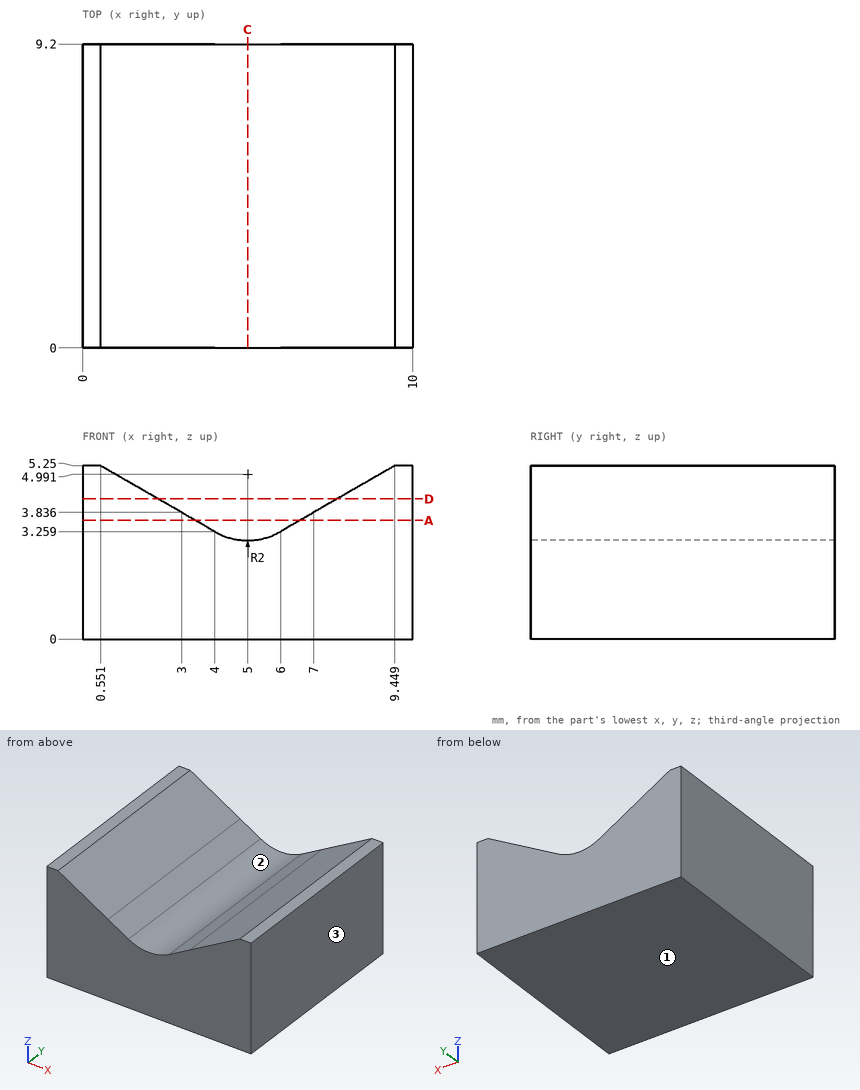
Design review of the part shown in the three views and the two pictorial views. Dimensions are in mm from the part's minimum x, y and z. Coordinates: 2 decimals unless noted, no trailing zeros. Write each loop counter-clockwise with the first axis right and the second up, starting at its lowest first coordinate (ties: lowest second). Pieces come first, ordered by that corner, then holes. Notation, with made-up numbers: (60, 9.5) - (69, 9.5) arc R23 cw to (69, 22.5) - close; hole circle Ø7 at (-12, 69). An arc over 180 degrees is marked (long way). Write item = value, one per line.
(1) Consider section D-D, the plane z = 4.25. Give the boundary of the cut face in (x, y).
Result sheet:
outline = (0, 0) - (2.28, 0) - (2.28, 9.2) - (0, 9.2) - close; (7.72, 0) - (10, 0) - (10, 9.2) - (7.72, 9.2) - close
(2) Consider section A-A, the plane z = 3.6. Give the boundary of the cut face in (x, y).
Result sheet:
outline = (0, 0) - (3.41, 0) - (3.41, 9.2) - (0, 9.2) - close; (6.59, 0) - (10, 0) - (10, 9.2) - (6.59, 9.2) - close
(3) For line 1 (Z direction, x = 5, y = 3.25); line 2 (X direction, y = 1.25, z = 3.4) (1 decimal); line 3 (X direction, y = 7, z = 4.1) (1 decimal), list the stretches that pass through material, from the lowest coordinate up. Write a range as [from, to].
Result sheet:
line_1 = [0, 2.99]
line_2 = [0, 3.8], [6.2, 10]
line_3 = [0, 2.5], [7.5, 10]
(4) Consider section C-C, the plane x = 5. Give the boundary of the cut face in (y, z).
Result sheet:
outline = (0, 0) - (9.2, 0) - (9.2, 2.99) - (0, 2.99) - close
(5) For P1, Ø2, axis at x = 2, z = 1.5, coming from the -Y side; P2, Ø1.5, axis at x = 2, y = 1.5, coming from the +Z side (1 decimal); P3, Ø1, axis at x = 5, y = 3.5, coming from the +Z side, all flat-tipped, find the tip position at first contact; note any pin that passes through.
Result sheet:
P1 = 0
P2 = 4.8
P3 = 3.05
(6) Mouldability with a two-part tool opening along X and no side actions: class the marked faces 1, 2 and 3 as pulls with the +X half, pulls with the -X half, needs draft (parallel to the pull), parting line crosses it, or undercut.
Result sheet:
face_1 = needs draft
face_2 = undercut
face_3 = pulls with the +X half
